Check sheet for the modelled part. Datum: model origin and axes. Units: mm. A direction names the side the tool comes from. Round coordinates to 2 decimals unless told otherwise and drop trailing zeros. Loops run counter-clockwise (first coordinate to the right, second up) from the corner with the lowest first, then second, coordinate; pieces in that order, holes last. Notation, with made-up numbers: (-30, 3.25) -> (18, 3.25) arc R23 cw to (18, 21.25) -> close; hole circle Ø4 at (-2, -40). An arc over 180 degrees is marked (long way). One line per question, with ' | ' between items.
```python
from build123d import *

# Parameters (mm, degrees)
SKETCH1_W           = 6
SKETCH1_H           = 6
SKETCH1_W_2         = 10
SKETCH1_H_2         = 5
BOSS_EXTRUDE1_DEPTH = 6


with BuildPart() as part:
    # Sketch1 → Boss-Extrude1 (new body)
    with BuildSketch(Plane(origin=(0, 0, 0), x_dir=(0, 0, -1), z_dir=(1, 0, 0))):
        Polygon((-15, 27.5), (15, 27.5), (15, -27.5), (9, -27.5), (9, -21.5), (3, -21.5), (3, -27.5), (-3, -27.5), (-3, -21.5), (-9, -21.5), (-9, -27.5), (-15, -27.5), align=None)
        with Locations((-6, 19.5)):
            Rectangle(SKETCH1_W, SKETCH1_H, mode=Mode.SUBTRACT)
        with Locations((6, 19.5)):
            Rectangle(SKETCH1_W, SKETCH1_H, mode=Mode.SUBTRACT)
        with Locations((0, 0.5)):
            Rectangle(SKETCH1_W_2, SKETCH1_H_2, mode=Mode.SUBTRACT)
    extrude(amount=BOSS_EXTRUDE1_DEPTH)


solid = part.part
```
(1) Sectioned sample at B-B, the plane x = 2.3. Record the cut outline in (y, z).
Answer:
outline: (-27.5, -15) -> (27.5, -15) -> (27.5, 15) -> (-27.5, 15) -> (-27.5, 9) -> (-21.5, 9) -> (-21.5, 3) -> (-27.5, 3) -> (-27.5, -3) -> (-21.5, -3) -> (-21.5, -9) -> (-27.5, -9) -> close; hole (-2, -5) -> (3, -5) -> (3, 5) -> (-2, 5) -> close; hole (16.5, -9) -> (22.5, -9) -> (22.5, -3) -> (16.5, -3) -> close; hole (16.5, 3) -> (22.5, 3) -> (22.5, 9) -> (16.5, 9) -> close
(2) Go/stop test with a flat-tipped pin: pin 1 (1.8 mm diameter, centred on x = 2.5, z = -5.5, fed in from -Y). Record where the tip stops, or that it passes through.
Answer:
pin 1: stops at y = -21.5
(3) Sectioned sample at A-A, the plane z = -7. Record the cut outline in (x, y), and give its area (3 significant figures).
Answer:
outline: (0, -21.5) -> (6, -21.5) -> (6, 16.5) -> (0, 16.5) -> close; (0, 22.5) -> (6, 22.5) -> (6, 27.5) -> (0, 27.5) -> close | area: 258 mm2
(4) Set-up check for faces 5 (the face through (3, -27.5, -12)), 6 (the face through (3, -25, 3)), 7 (the face through (3, 22.5, 6)): record each of +Z, -Z, +X, -X, +Y, -Y from which the full face is reachable in a straight line by a thin tool's end or side.
Answer:
face 5: +Z, -Z, +X, -X, -Y | face 6: +X, -X, -Y | face 7: +X, -X
(5) Scan lines: probe 1 along Z at (x, y) = (1.15, 17); probe 2 along Y at (x, z) = (2.9, -7); probe 3 along Y at (x, z) = (1.7, 0). Record each from-to range of solid material in increasing order.
Answer:
probe 1: z = -15 to -9, -3 to 3, 9 to 15 | probe 2: y = -21.5 to 16.5, 22.5 to 27.5 | probe 3: y = -27.5 to -2, 3 to 27.5
(6) Mould release check, pull along Y, two halves, no side actions. Record for faces 1 (the face through (0, 6, 0)), 2 (the face through (3, 19, 3)), 3 (the face through (3, -21.5, -6)), 4 (the face through (3, -2, 0)): +Y half, -Y half, draft (parallel to the pull), parting line (faces both ways), or undercut.
Answer:
face 1: draft | face 2: undercut | face 3: -Y half | face 4: undercut
